Read the model definition and answer for the solid it produces. Units are mm, in the model's axes. A direction names the side the tool comes from. Coordinates: 2 decimals unless noted, no trailing zeros. Order: outer loops, then holes, each group sorted by start corner. A loop starts at its lowest first (then second) coordinate and runs counter-clockwise, first axis right, second up. Notation, with made-up numbers: M 39.5,12.25 L 86.5,12.25 A33 ccw 86.5,44.25 Z; hole C -25.75,-10 d2. An arc over 180 degrees is marked long. Use a Markdown table: item, result. Add a question column.
1) For faces 1 (the face through (-2.24, 17.43, 3.46)), 2 (the face through (0.54, 13.26, 2.48)), determine the directions among +Z, -Z, +X, -X, +Y, -Y from which every point of the face is accessible in a straight line to the end or side of a thin tool.
2) Find section D-D on y = 9.5. Write down the section's boundary in (x, z), plus the area to 3 significant figures.
3) Find section A-A on y = 0. Write down the section's boundary in (x, z), plus the area to 3 significant figures.
4) Find the intervals of material crossed by probe 1 along Y at (x, z) = (0, 4.8); probe 2 along Y at (x, z) = (1.5, 3.75); probe 3 along Y at (x, z) = (0, 1.95), in increasing order. Write a range as [from, to].
5) Each of these flat-tipped pins is pushed along its axis until it touches: pin 1 Ø1.5 at (x, y) = (1, 1) entering from -Z; pin 2 Ø1 at (x, z) = (-2, 2.5) entering from -Y; pin 3 Ø1.7 at (x, y) = (0, 15.6) entering from -Z. Where does it stop, or does it pass through?
6) The mould has two halves that part along Y. Classify faces 3 (the face through (1, -0.32, 4.99)), 4 (the face through (-3.587, 1.814, 2.915)), 5 (the face through (-2.099, 7.993, 5.816)): released by +Y, released by -Y, zero draft, split by the parting line, or undercut.
7) Find section B-B on x = 0.5. Write down the section's boundary in (y, z), plus the area to 3 significant figures.
8) Find section C-C on z = 2.45. Write down the section's boundary in (x, y), plus the area to 3 significant figures.
Autodesk Inventor part; units mm, degrees
ref_plane "Arbeitsebene1" through (0, 7.8495, 6) normal (0, 1, 0) x (1, 0, 0)
ref_plane "YZ Plane" through (0, 0, 0) normal (1, 0, 0) x (0, 1, 0)
ref_plane "XZ Plane" through (0, 0, 0) normal (0, 1, 0) x (-1, 0, 0)
sketch "Skizze1" plane through (0, 0, 0) normal (0, 0, 1) x (1, 0, 0)
  circle A0 centre (0, 0) radius 2
  circle A1 centre (0, 0) radius 1.05
  circle A2 centre (0, 15.5995) radius 2
  circle A3 centre (0, 15.5995) radius 1.05
  line L0 (0, 18.5995) -> (4, 18.5995)
  line L1 (-2.8284, 15.7711) -> (0, 18.5995)
  arc A4 (-2.8284, 15.7711) -> (-4, 12.9427) centre (0, 12.9427) ccw
  line L2 (-4, 12.9427) -> (-4, 10.689)
  line L3 (-4, 5.0101) -> (-4, 2.7564)
  arc A5 (-4, 2.7564) -> (-2.8284, -0.072) centre (0, 2.7564) ccw
  line L4 (0, -2.9005) -> (-2.8284, -0.072)
  line L5 (4, -2.9005) -> (0, -2.9005)
  line L6 (4, 18.5995) -> (4, -2.9005)
  line L7 (-4, 10.689) -> (-4, 5.0101)
  point P0 (0, 0)
extrude "Extrusion1" add sketch "Skizze1" along normal blind 4 contours L0 L6 L5 L4 A5 L3 L7 L2 A4 L1
sketch "Skizze2" plane through (0, 0, 4) normal (0, 0, 1) x (1, 0, 0)
  line L0 (0, 18.5995) -> (-2.8284, 15.7711)
  arc A0 (-2.8284, 15.7711) -> (-4, 12.9427) centre (0, 12.9427) ccw
  line L1 (-4, 12.9427) -> (-4, 2.7564)
  arc A1 (-4, 2.7564) -> (-2.8284, -0.072) centre (0, 2.7564) ccw
  line L2 (-2.8284, -0.072) -> (0, -2.9005)
  line L3 (0, -2.9005) -> (4, -2.9005)
  line L4 (4, -2.9005) -> (4, 18.5995)
  line L5 (4, 18.5995) -> (0, 18.5995)
  circle A2 centre (0, 15.5995) radius 2
  circle A3 centre (0, 0) radius 2
  circle A4 centre (0, 15.5995) radius 1.05
  circle A5 centre (0, 0) radius 1.05
  point P0 (0, 0)
  dimension "d2" = 2.1
  dimension "d3" = 2.1
extrude "Extrusion2" add sketch "Skizze2" along normal blind 2 contours L5 L4 L3 L2 A1 L1 A0 L0 | A2 | A3
sketch "Skizze3" plane through (0, 0, 0) normal (0, 0, -1) x (-1, 0, 0)
  line L0 (0, -2.9005) -> (-4, -2.9005)
  line L1 (-4, -2.9005) -> (-4, 7.8495)
  line L2 (-4, -2.9005) -> (-4, 18.5995)
  line L3 (-4, 7.8495) -> (1, 7.8495)
  circle A0 centre (1, 7.8495) radius 4.25
  line L4 (1, 7.8495) -> (5.25, 7.8495)
  line L5 (4, 12.9427) -> (4, 2.7564)
  point P0 (0, 0)
  point P1 (4, 7.8495)
  point P2 (4, 10.8599)
  point P3 (-3.25, 7.8495)
  dimension "d7" = 8.5
  dimension "d8" = 3
revolve "Umdrehung1" cut sketch "Skizze3" angle 360 about axis through (4, 7.8495, 0) along (-1, 0, 0) picked at (3, 8.853) contours A0 L5 L4 L3
sketch "Skizze4" plane through (0, 0, 0) normal (0, 0, -1) x (-1, 0, 0)
  line L0 (-4.7683, -3.7941) -> (5.6191, -3.7941)
  line L1 (5.6191, -3.7941) -> (5.6191, 20.4958)
  line L2 (5.6191, 20.4958) -> (-4.7683, 20.4958)
  line L3 (-4.7683, 20.4958) -> (-4.7683, -3.7941)
  point P0 (0, 0)
extrude "Extrusion3" cut sketch "Skizze4" against normal blind 1
sketch "Skizze5" plane through (4, -2.9005, 6) normal (1, 0, 0) x (0, 0, -1)
  line L0 (5, 0) -> (5, 21.5)
  line L1 (5, 21.5) -> (0, 21.5)
  line L2 (0, 0) -> (0, 21.5)
  line L3 (5, 0) -> (0, 0)
  point P0 (6, 2.9005)
extrude "Extrusion4" cut sketch "Skizze5" against normal blind 1
sketch "Skizze6" plane through (0, 0, 1) normal (0, 0, -1) x (-1, 0, 0)
  line L0 (2.8284, -0.072) -> (0, -2.9005)
  line L1 (0, -2.9005) -> (0.4894, -2.9005)
  arc A0 (2.8284, -0.072) -> (4, 2.7564) centre (0, 2.7564) ccw
  line L2 (0.4894, -2.9005) -> (4, -2.9005)
  line L3 (4, -2.9005) -> (4, 2.7564)
  point P0 (0, 0)
  point P1 (3.7092, 1.2591)
extrude "Extrusion5" add sketch "Skizze6" against normal up to surface (5 mm away)
ref_plane "Arbeitsebene1" through (0, 7.8495, 6) normal (0, 1, 0) x (1, 0, 0)
sketch "Skizze9" plane through (0, 0, 1) normal (0, 0, -1) x (-1, 0, 0)
  circle A0 centre (0, 0) radius 2.5
  dimension "d24" = 5
extrude "Extrusion8" cut sketch "Skizze9" against normal up to surface (3 mm away)
sketch "Skizze10" plane through (0, 0, 1) normal (0, 0, -1) x (-1, 0, 0)
  line L0 (0.6938, -3.6003) -> (3.1846, -0.5858)
  line L1 (3.1846, -0.5858) -> (4, 4.2826)
  line L2 (4, -2.9005) -> (4, 5.0101)
  line L3 (4, -2.9005) -> (-3, -2.9005)
  point P0 (0, 0)
  point P1 (1.272, -2.9005)
extrude "Extrusion9" cut sketch "Skizze10" against normal through all
mirror "Spiegeln3" about plane through (0, 7.8495, 6) normal (0, 1, 0) of "Extrusion5", "Extrusion8", "Extrusion9"
sketch "Skizze11" plane through (3, 18.5995, 6) normal (0, 1, 0) x (1, 0, 0)
  line L0 (-7, 2.9896) -> (-7, 5)
  line L1 (-7.4841, 2.5704) -> (-4.5207, -0.7469)
  line L2 (-4.5207, -0.7469) -> (-5.1252, -3.6367)
  line L3 (-5.1252, -3.6367) -> (-9.8579, -0.57)
  line L4 (-9.8579, -0.57) -> (-7.4841, 2.5704)
  point P0 (-3, 6)
extrude "Extrusion10" cut sketch "Skizze11" against normal through all
chamfer "Fase2" distance 0.5 angle 45 1 edges at (-2.188, 7.8495, 6)
properties part number "BallJointClamp"
Check result:
| question | item | result |
|---|---|---|
| 1 | face 1 | +Z, -Z, -X, +Y |
| 1 | face 2 | -Z |
| 2 | outline | M -4,2.52 A3.92 cw 2.79,1 L 3,1 L 3,6 L -1.69,6 L -2.52,5.63 L -4,3.97 Z |
| 2 | area | 17.4 mm2 |
| 3 | outline | M -3.28,1 L -2.5,1 L -2.5,4 L -1.05,4 L -1.05,6 L -1.69,6 L -2.52,5.63 L -3.28,4.77 Z; M 1.05,4 L 2.5,4 L 2.5,1 L 3,1 L 3,6 L 1.05,6 Z |
| 3 | area | 11.4 mm2 |
| 4 | probe 1 | y = [-2.9, -1.05], [1.05, 14.55], [16.65, 18.6] |
| 4 | probe 2 | y = [-2.9, -2], [2, 13.7], [17.7, 18.6] |
| 4 | probe 3 | y = [-2.9, -2.5], [2.5, 4.21], [11.49, 13.2], [18.2, 18.6] |
| 5 | pin 1 | stops at z = 4 |
| 5 | pin 2 | stops at y = -2.62 |
| 5 | pin 3 | passes through |
| 6 | face 3 | undercut |
| 6 | face 4 | released by -Y |
| 6 | face 5 | zero draft |
| 7 | outline | M -2.9,1 L -2.45,1 L -2.45,4 L -0.92,4 L -0.92,6 L -2.9,6 Z; M 0.92,4 L 2.45,4 L 2.45,1 L 4,1 A3.98 cw 11.7,1 L 13.25,1 L 13.25,4 L 14.68,4 L 14.68,6 L 0.92,6 Z; M 16.52,4 L 18.15,4 L 18.15,1 L 18.6,1 L 18.6,6 L 16.52,6 Z |
| 7 | area | 53.7 mm2 |
| 8 | outline | M -4,4.28 L -3.18,-0.59 L -1.27,-2.9 L 3,-2.9 L 3,18.6 L -1.27,18.6 L -3.18,16.28 L -4,11.42 L -4,9.6 A3.47 cw long -4,6.1 Z; hole C 0,0 d5; hole C 0,15.7 d5 |
| 8 | area | 62.3 mm2 |
